```python
from build123d import *

# Parameters (mm, degrees)
CROQUIS1_W                 = 23
CROQUIS1_H                 = 6
CROQUIS1_R                 = 1.5
SALIENTE_EXTRUIR1_DEPTH    = 3
RECUBRIR1_DEPTH            = 23
CROQUIS2_R                 = 1.5
CORTAR_EXTRUIR1_DEPTH      = 3
CROQUIS3_R                 = 34.0625
CORTAR_EXTRUIR2_DEPTH      = 14
SALIENTE_EXTRUIR2_DEPTH    = 2
SALIENTE_EXTRUIR3_DEPTH    = 2
CROQUIS8_W                 = 11.736
CROQUIS8_H                 = 2
SALIENTE_EXTRUIR4_DEPTH    = 2
CORTAR_EXTRUIR3_REACH      = 33.064
CORTAR_EXTRUIR3_END_RADIUS = 34.0625


# Read off the part's stored shape, not the designer's step: Recubrir1
with BuildPart() as part:
    # Croquis1 → Saliente-Extruir1 (new body)
    with BuildSketch(Plane.XY):
        with Locations((11.5, 3)):
            Rectangle(CROQUIS1_W, CROQUIS1_H)
        with Locations((4, 3)):
            Circle(CROQUIS1_R, mode=Mode.SUBTRACT)
        with Locations((19, 3)):
            Circle(CROQUIS1_R, mode=Mode.SUBTRACT)
    extrude(amount=SALIENTE_EXTRUIR1_DEPTH)

    # Recubrir1 outline → Recubrir1 (add)
    with BuildSketch(Plane.YZ):
        Polygon((3, 3), (20, 3), (20, 6), (6, 6), align=None)
    extrude(amount=RECUBRIR1_DEPTH)

    # Croquis2 → Cortar-Extruir1 (cut)
    with BuildSketch(Plane.XY.offset(3)):
        with Locations((4, 3)):
            Circle(CROQUIS2_R)
        with Locations((19, 3)):
            Circle(CROQUIS2_R)
    extrude(amount=CORTAR_EXTRUIR1_DEPTH, mode=Mode.SUBTRACT)

    # Croquis3 → Cortar-Extruir2 (cut)
    with BuildSketch(Plane(origin=(0, 20, 0), x_dir=(1, 0, 0), z_dir=(0, 1, 0))):
        with Locations((11.5, 29.0625)):
            Circle(CROQUIS3_R)
    extrude(amount=-CORTAR_EXTRUIR2_DEPTH, mode=Mode.SUBTRACT)

    # Croquis6 → Saliente-Extruir2 (add)
    with BuildSketch(Plane(origin=(0, 20, 0), x_dir=(1, 0, 0), z_dir=(0, 1, 0))):
        Polygon((22.5, -6), (0.5, -6), (0.5, -8), (1.967, -9), (1.967, -8), (3.434, -9), (3.434, -8), (4.901, -9), (4.901, -8), (6.368, -9), (6.368, -8), (7.835, -9), (7.835, -8), (9.302, -9), (9.302, -8), (10.769, -9), (10.769, -8), (12.236, -9), (12.236, -8), (13.703, -9), (13.703, -8), (15.17, -9), (15.17, -8), (16.637, -9), (16.637, -8), (18.104, -9), (18.104, -8), (19.571, -9), (19.571, -8), (21.038, -9), (21.038, -8), (22.5, -9), align=None)
    extrude(amount=-SALIENTE_EXTRUIR2_DEPTH)

    # Croquis7 → Saliente-Extruir3 (add)
    with BuildSketch(Plane(origin=(0, 15.767364365, 0), x_dir=(1, 0, 0), z_dir=(0, 1, 0))):
        Polygon((18.099, -9), (18.099, -8), (19.566, -9), (19.566, -8), (21.033, -9), (21.033, -8), (22.5, -9), (22.5, -6), (16.632, -6), (16.632, -8), align=None)
    extrude(amount=-SALIENTE_EXTRUIR3_DEPTH)

    # Croquis8 → Saliente-Extruir4 (add)
    with BuildSketch(Plane(origin=(0, 12.767364365, 0), x_dir=(1, 0, 0), z_dir=(0, 1, 0))):
        with Locations((16.632, -7)):
            Rectangle(CROQUIS8_W, CROQUIS8_H)
        Polygon((15.165, -8), (13.698, -8), (15.165, -9), align=None)
        Polygon((13.698, -8), (12.231, -8), (13.698, -9), align=None)
        Polygon((12.231, -8), (10.764, -8), (12.231, -9), align=None)
        Polygon((16.632, -9), (16.632, -8), (15.165, -8), align=None)
        Polygon((18.099, -9), (18.099, -8), (16.632, -8), align=None)
        Polygon((19.566, -9), (19.566, -8), (18.099, -8), align=None)
        Polygon((21.033, -9), (21.033, -8), (19.566, -8), align=None)
        Polygon((22.5, -9), (22.5, -8), (21.033, -8), align=None)
    extrude(amount=-SALIENTE_EXTRUIR4_DEPTH)

    # Cortar-Extruir3: up to this cylinder (the profile starts outside it)
    cortar_extruir3_end = Plane(origin=(11.5, 15.383682, -29.0625), z_dir=(0, 1, 0)) * Cylinder(CORTAR_EXTRUIR3_END_RADIUS, 135.253, mode=Mode.PRIVATE)
    # Croquis9 → Cortar-Extruir3 (cut, up to the surface)
    with BuildSketch(Plane.XY.offset(6), mode=Mode.PRIVATE) as cortar_extruir3_sk1:
        Polygon((10.764, 12.767364365), (16.632, 12.767364365), (16.632, 13.767364365), (16.632, 15.767364365), (16.632, 18), (6, 18), (6, 12.767364365), align=None)
    cortar_extruir3_tool1 = extrude(cortar_extruir3_sk1.sketch, amount=-CORTAR_EXTRUIR3_REACH, mode=Mode.PRIVATE) - cortar_extruir3_end
    add(cortar_extruir3_tool1.solids().sort_by_distance((11.316, 15.383682, 6))[0], mode=Mode.SUBTRACT)


solid = part.part
```
For this review, take the finished solid that the model builds, in its own axes (mm). A direction names the side the tool comes from. Coordinates: 2 decimals unless noted, no trailing zeros. Write each loop counter-clockwise with the first axis right and the second up, starting at its lowest first coordinate (ties: lowest second). Pieces come first, ordered by that corner, then holes.
(1) Wall thickness on probe 1 along Y at (x, z) = (22.25, 7); probe 2 along Y at (x, z) = (4, 2.65); probe 3 along Y at (x, z) = (14.5, 5): over which ranges is each line inside the solid? List them lowest first.
(2) For pin 1 Ø1.5 at (x, y) = (15, 4.5) entering from +Z; pin 2 Ø0.8 at (y, z) = (11.5, 8.5) entering from +X; pin 3 Ø3.5 at (x, y) = (8.5, 2) entering from +Z, all flat-tipped, find the tip position at first contact; note any pin that passes through.
(3) Add section A-A on z = 7. Give the boundary of the cut face in (x, y), then the cut area to 3 significant figures.
(4) Add section C-C on x = 19. Give the boundary of the cut face in (y, z).
(5) Add section D-D on z = 1.75. Give the boundary of the cut face in (x, y), then the cut area to 3 significant figures.
(6) Tool access review of faces 1 (the face through (8.558, 19.014, 8.493)), 2 (the face through (6, 15, 5)), 3 (the face through (11, 18, 7)), 4 (the face through (22.5, 12, 8)): name each direction out of +Z, -Z, +X, -X, +Y, -Y from which nothing blocks a thin tool from reaching the whole face with its end or side.
(7) Add section B-B on y = 15. Give the boundary of the cut face in (x, z) (1 decimal), then the cut area to 3 significant figures.
(8) The part is to be moulded in two halves that separate along Y. For faces 5 (the face through (11, 20, 7)), 6 (the face through (0.5, 19, 7)), 7 (the face through (20, 13.767, 7)), say which applies: +Y half, -Y half, draft (parallel to the pull), parting line (faces both ways), or undercut.
Answer sheet:
1. probe 1: y = 10.77 to 12.77, 13.77 to 15.77, 18 to 20
1. probe 2: y = 0 to 1.5, 4.5 to 6
1. probe 3: y = 5 to 12.77, 18 to 20
2. pin 1: stops at z = 5.25
2. pin 2: stops at x = 22.5
2. pin 3: stops at z = 3.75
3. outline: (0.5, 18) - (22.5, 18) - (22.5, 20) - (0.5, 20) - close; (10.76, 10.77) - (22.5, 10.77) - (22.5, 12.77) - (10.76, 12.77) - close; (16.63, 13.77) - (22.5, 13.77) - (22.5, 15.77) - (16.63, 15.77) - close
3. area: 79.2 mm2
4. outline: (0, 0) - (1.5, 0) - (1.5, 3) - (0, 3) - close; (4.5, 0) - (6, 0) - (6, 4.16) - (20, 4.16) - (20, 8.61) - (18, 8.61) - (18, 6) - (15.77, 6) - (15.77, 8.61) - (13.77, 8.61) - (13.77, 6) - (12.77, 6) - (12.77, 8.61) - (10.77, 8.61) - (10.77, 6) - (6, 6) - (4.5, 4.5) - close
5. outline: (0, 0) - (23, 0) - (23, 6) - (0, 6) - close; hole circle Ø3 at (4, 3); hole circle Ø3 at (19, 3)
5. area: 124 mm2
6. face 1: +Z, +Y, -Y
6. face 2: +Z, -Z
6. face 3: +Z
6. face 4: +Z, +X, +Y, -Y
7. outline: (0, 3) arc R34.1 cw to (6, 4.6) - (6, 6) - (0, 6) - close; (16.6, 4.6) arc R34.1 cw to (23, 3) - (23, 6) - (22.5, 6) - (22.5, 9) - (21, 8) - (21, 9) - (19.6, 8) - (19.6, 9) - (18.1, 8) - (18.1, 9) - (16.6, 8) - close
7. area: 40.7 mm2
8. face 5: +Y half
8. face 6: draft
8. face 7: undercut
